Check sheet for the drawn part. Datum: minimum x, y, z corner. Units: mm. A direction names the side the tool comes from. Give positions to 0.01 mm unless a question says otherwise; leave off trailing zeros. Write each loop counter-clockwise with the first axis right and the second up, starting at its lowest first coordinate (ties: lowest second). Pieces come first, ordered by that corner, then holes. Notation, with made-up numbers: M 88,-28.75 L 99,-28.75 A20 cw 99,0.25 Z; hole C 0,-12.5 d5. An arc over 180 degrees is marked long. Write item = value, one per line. Start each with the question number.
1) Gauge pin test, flat ends, axial feed: pin 1 (1.5 mm diameter, centred on x = 3.5, z = 1.5, fed in from +Y); pin 2 (2 mm diameter, centred on x = 2.5, y = 3, fed in from -Z). Record the tip position at first contact, or that the pin passes through.
2) Set-up check for the marked faces 1 and 2: record each of +Z, -Z, +X, -X, +Y, -Y from which the full face is reachable in a straight line by a thin tool's end or side.
3) Sectioned sample at B-B, the plane y = 0.8. Record the cut outline in (x, z).
4) Scan lines: L1, parallel to Y at x = 5.2, z = 2.8; L2, parallel to X at y = 0.3, z = 2.6; L3, parallel to Z at x = 4.45, y = 0.45. Record each from-to range of solid material in increasing order.
5) Sectioned sample at A-A, the plane y = 2.3. Record the cut outline in (x, z).
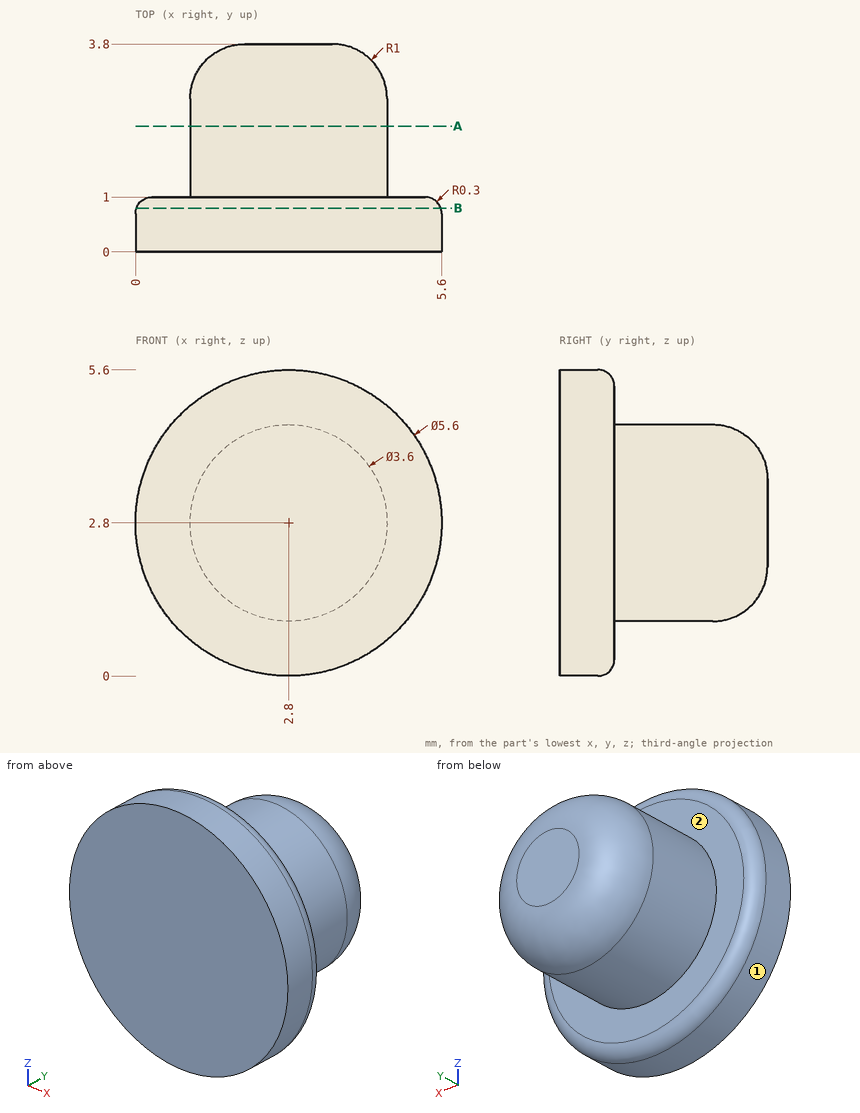
Data:
q1.pin_1 = 3.8
q1.pin_2 = 1
q2.face_1 = +Y, -Y
q2.face_2 = +Y
q3.outline = C 2.8,2.8 d5.57
q4.L1 = 0 to 1
q4.L2 = 0.01 to 5.59
q4.L3 = 0.54 to 5.06
q5.outline = C 2.8,2.8 d3.6
